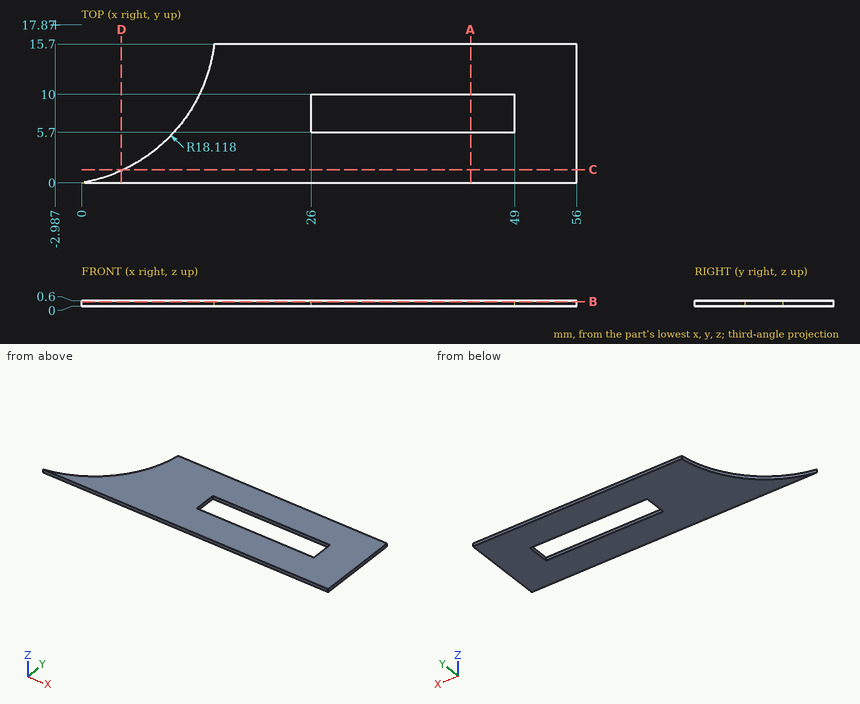
Input: dimensioned drawing with shaded views. Units: mm. Origin: part minimum x, y, z. Round coordinates to 2 decimals unless told otherwise and drop trailing zeros. Write each loop counter-clockwise with the first axis right and the second up, starting at its lowest first coordinate (ties: lowest second). Pieces come first, ordered by that corner, then holes. Notation, with made-up numbers: (49.25, -3) - (73.25, -3) arc R12 cw to (73.25, 5) - close; hole circle Ø3 at (31, 15). An arc over 180 degrees is marked (long way). Write item = value, one per line.
(1) Section query B-B on z = 0.5. Output: boundary loops of the cut face in (x, y) (1 decimal).
Geometry check:
outline = (0, 0) - (56, 0) - (56, 15.7) - (15, 15.7) arc R18.1 cw to start; hole (26, 5.7) - (49, 5.7) - (49, 10) - (26, 10) - close
(2) Section query A-A on x = 44. Output: boundary loops of the cut face in (y, z).
Geometry check:
outline = (0, 0) - (5.7, 0) - (5.7, 0.6) - (0, 0.6) - close; (10, 0) - (15.7, 0) - (15.7, 0.6) - (10, 0.6) - close
(3) Material intervals for probe 1 along Y at (x, z) = (37.5, 0.1); probe 2 along X at (y, z) = (6.5, 0.2); probe 3 along X at (y, z) = (5.5, 0.3), sorted ascending.
Geometry check:
probe_1 = 0 to 5.7, 10 to 15.7
probe_2 = 11.12 to 26, 49 to 56
probe_3 = 10.25 to 56
(4) Section query D-D on x = 4.5. Output: boundary loops of the cut face in (y, z).
Geometry check:
outline = (0, 0) - (1.37, 0) - (1.37, 0.6) - (0, 0.6) - close
(5) Section query C-C on y = 1.5. Output: boundary loops of the cut face in (x, z).
Geometry check:
outline = (4.78, 0) - (56, 0) - (56, 0.6) - (4.78, 0.6) - close
